Answer from the drawing. Dimensions are ordinates in mm from the lowest x, y and z of the part. Round coordinates to 2 decimals unless told otherwise and drop trailing zeros. Write each loop counter-clockwise with the first axis right and the second up, starting at its lowest first coordinate (ties: lowest second). Pieces come first, ordered by that corner, then holes. Notation, with made-up numbers: M -40,-32.75 L -20,-32.75 A13 cw -20,-19.75 Z; hole C 33,36 d3. An arc over 180 degrees is marked long. Answer as CSV lines item,"result". Start each with the question number.
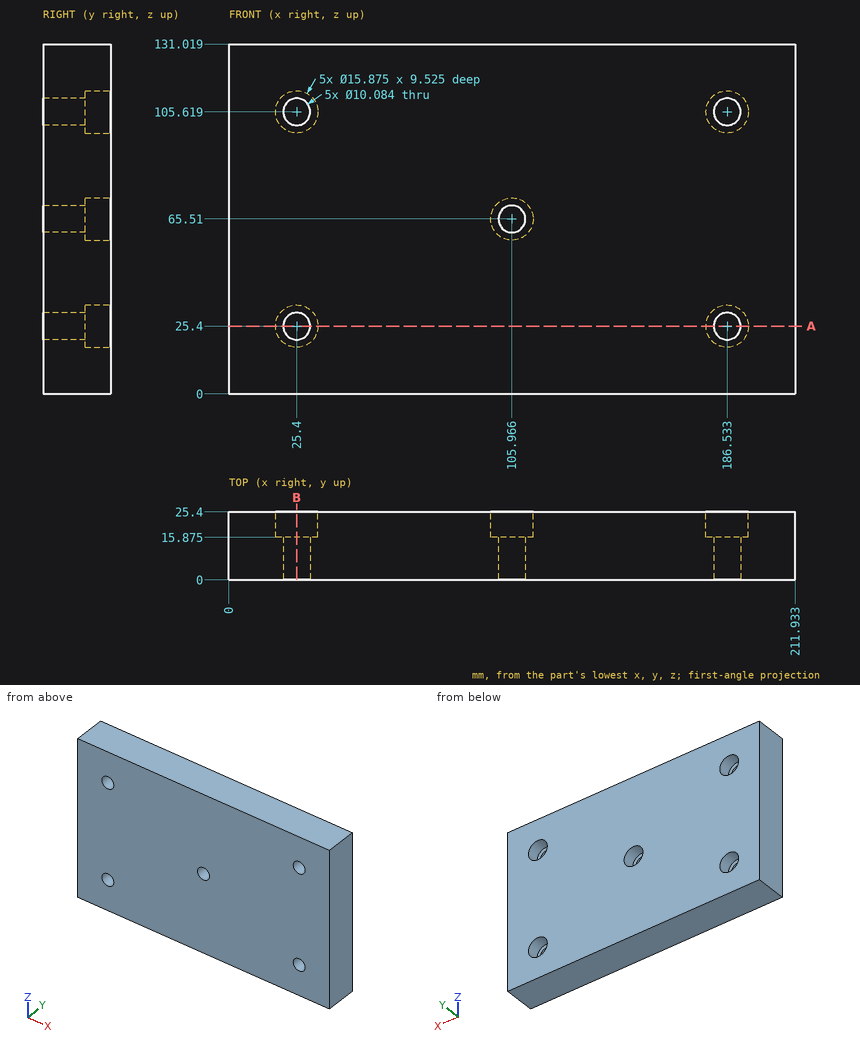
Q1. This flat-tipped pin is pushed along its axis until it touches: P1, Ø8, axis at x = 104.5, z = 68.5, coming from the +Y side (1 decimal). Where does it stop, or does it pass through?
Q2. Find section B-B (x = 25.4). Determine the outline of the cut face in (y, z) (1 decimal).
Q3. Find section A-A (z = 25.4). Determine the outline of the cut face in (x, y) (1 decimal), plus the area to 3 significant figures.
Q4. Straight lines are drawn through the part: L1, parallel to Z at x = 25.4, y = 18.25; L2, parallel to Z at x = 25, y = 13 (1 decimal); L3, parallel to X at y = 23, z = 21 (1 decimal). For each, find the intervals that lie inside material, in ascending order.
Reported:
1,P1,"stops at y = 15.9"
2,outline,"M 0,0 L 25.4,0 L 25.4,17.5 L 15.9,17.5 L 15.9,20.4 L 0,20.4 Z; M 0,30.4 L 15.9,30.4 L 15.9,33.3 L 25.4,33.3 L 25.4,97.7 L 15.9,97.7 L 15.9,100.6 L 0,100.6 Z; M 0,110.7 L 15.9,110.7 L 15.9,113.6 L 25.4,113.6 L 25.4,131 L 0,131 Z"
3,outline,"M 0,0 L 20.4,0 L 20.4,15.9 L 17.5,15.9 L 17.5,25.4 L 0,25.4 Z; M 30.4,0 L 181.5,0 L 181.5,15.9 L 178.6,15.9 L 178.6,25.4 L 33.3,25.4 L 33.3,15.9 L 30.4,15.9 Z; M 191.6,0 L 211.9,0 L 211.9,25.4 L 194.5,25.4 L 194.5,15.9 L 191.6,15.9 Z"
3,area,"4,760 mm2"
4,L1,"z = 0 to 17.46, 33.34 to 97.68, 113.56 to 131.02"
4,L2,"z = 0 to 20.4, 30.4 to 100.6, 110.6 to 131"
4,L3,"x = 0 to 18.8, 32 to 179.9, 193.1 to 211.9"
